Input: part model. Units: mm. Frame: model coordinates. Face numbers are marked on the shaded views. A direction names the side the tool comes from. Round coordinates to 2 decimals unless told otherwise and drop trailing zeros. Loops run counter-clockwise (first coordinate to the right, second up) from the corner with the lowest first, then second, coordinate; pieces in that order, holes last. Notation, with made-up numbers: (85, -12.75) - (124, -12.75) arc R22 ccw to (124, -2.75) - close; hole circle Ø9 at (87, 66.5). An arc over 180 degrees is marked (long way). Use CSV: the item, a comma, the result in double quotes. Start each with the question number.
1. Pin query (flat end, axial travel): P1, Ø6, axis at y = 102.5, z = 18, coming from the -X side; P2, Ø6, axis at x = 159.5, z = 30, coming from the +Y side; P3, Ø3, axis at y = 127, z = 28.5, coming from the +X side. Return the tip coordinate at first contact, or that it passes through.
2. Material intervals for probe 1 along Y at (x, z) = (156, 10); probe 2 along Z at (x, y) = (61, 215); probe 3 along X at (y, z) = (67.5, 6), sorted ascending. Write a range as from..to.
3. Access query for the marked faces 1, 2, 3 and 4. Directions: +Z, -Z, +X, -X, +Y, -Y. A direction counts if a zero-diameter tool reaches every point of the face in a straight line with its end or side. Return the directions, or none.
4. Cut plane D-D (x = 97.5). Return loops of the section in (y, z).
5. Cut plane A-A (z = 59). Return loops of the section in (x, y), and give its area (3 significant figures).
6. Cut plane B-B (x = 172.5). Return loops of the section in (y, z).
7. Cut plane C-C (y = 156). Return loops of the section in (x, z), and give its area (3 significant figures).
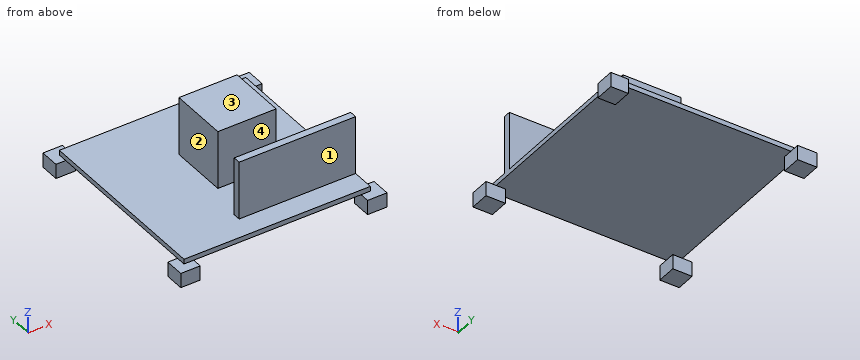
```python
from build123d import *

# Parameters (mm, degrees)
F0_W     = 243.84
F0_H     = 243.84
F1_DEPTH = 6.35
F2_W     = 76.2
F2_H     = 76.2
F3_DEPTH = 76.2
F4_W     = 12.7000009538
F4_H     = 12.7
F4_W_2   = 12.1249086118
F4_H_2   = 12.346994652
F4_W_3   = 9.7286785974
F5_DEPTH = 19.05
F6_W     = 152.4
F6_H     = 9.525
F7_DEPTH = 76.2


with BuildPart() as f1:
    # F0 (on Top) → F1 (new body)
    with BuildSketch(Plane.XY):
        with Locations((121.92, 121.92)):
            Rectangle(F0_W, F0_H)
    extrude(amount=F1_DEPTH)

    # F2 (on face) → F3 (join)
    with BuildSketch(Plane.XY.offset(6.35)):
        with Locations((141.9095646479, 127.1040961146)):
            Rectangle(F2_W, F2_H)
    extrude(amount=F3_DEPTH)

    # F4 (on face) → F5 (join)
    with BuildSketch(Plane(origin=(0, 0, 0), x_dir=(1, 0, 0), z_dir=(0, 0, -1))):
        Polygon((12.7000009538, 12.7), (-12.7, 12.7), (-12.7, -12.7), (0, -12.7), (0, 0), (12.7000009538, 0), align=None)
        with Locations((6.3500004769, -6.35)):
            Rectangle(F4_W, F4_H)
        Polygon((231.7150913882, 12.7), (231.7150913882, 0), (243.84, 0), (243.84, -12.7), (257.115092342, -12.7), (257.115092342, 12.7), align=None)
        with Locations((237.7775456941, -6.35)):
            Rectangle(F4_W_2, F4_H)
        with Locations((6.3500004769, -237.666502674)):
            Rectangle(F4_W, F4_H_2)
        Polygon((0, -243.84), (0, -231.493005348), (-12.7, -231.493005348), (-12.7, -256.893005348), (12.7000009538, -256.893005348), (12.7000009538, -243.84), align=None)
        Polygon((257.115092342, -231.493005348), (243.84, -231.493005348), (243.84, -243.84), (234.1113214026, -243.84), (234.1113214026, -256.893005348), (257.115092342, -256.893005348), align=None)
        with Locations((238.9756607013, -237.666502674)):
            Rectangle(F4_W_3, F4_H_2)
    extrude(amount=F5_DEPTH)

    # F6 (on face) → F7 (join)
    with BuildSketch(Plane.XY.offset(6.35)):
        with Locations((167.64, 33.6779164493)):
            Rectangle(F6_W, F6_H)
    extrude(amount=F7_DEPTH)


solid = f1.part
```
Established:
1,P1,"stops at x = 103.81"
1,P2,"stops at y = 165.2"
1,P3,"stops at x = 180.01"
2,probe 1,"y = 28.92..38.44, 89..165.2"
2,probe 2,"z = 0..6.35"
2,probe 3,"x = 0..243.84"
3,face 1,"+Z, +X, -X, -Y"
3,face 2,"+Z, -X, +Y"
3,face 3,"+Z, +X, -X, +Y, -Y"
3,face 4,"+Z, +X, -X"
4,outline,"(0, 0) - (243.84, 0) - (243.84, 6.35) - (38.44, 6.35) - (38.44, 82.55) - (28.92, 82.55) - (28.92, 6.35) - (0, 6.35) - close"
5,outline,"(91.44, 28.92) - (243.84, 28.92) - (243.84, 38.44) - (91.44, 38.44) - close; (103.81, 89) - (180.01, 89) - (180.01, 165.2) - (103.81, 165.2) - close"
5,area,"7,260 mm2"
6,outline,"(0, 0) - (243.84, 0) - (243.84, 6.35) - (165.2, 6.35) - (165.2, 82.55) - (89, 82.55) - (89, 6.35) - (38.44, 6.35) - (38.44, 82.55) - (28.92, 82.55) - (28.92, 6.35) - (0, 6.35) - close"
7,outline,"(0, 0) - (243.84, 0) - (243.84, 6.35) - (180.01, 6.35) - (180.01, 82.55) - (103.81, 82.55) - (103.81, 6.35) - (0, 6.35) - close"
7,area,"7,350 mm2"
